Verification items for the finished model (mm, model axes). Give positions to 0.01 mm unless a question says otherwise; leave off trailing zeros. Loops run counter-clockwise (first coordinate to the right, second up) from the corner with the lowest first, then second, coordinate; pieces in that order, holes last. Notation, with made-up numbers: M -18,-5.75 L 16,-5.75 A11 ccw 16,1.25 Z; hole C 28,-8 d2. An arc over 180 degrees is marked long. Write each question's results on one line, items separated by ' | '. Start each with the question number.
```python
from build123d import *

# Parameters (mm, degrees)
F0_W     = 100
F0_H     = 200
F0_R     = 5.1
F0_W_2   = 70
F0_H_2   = 110
F0_H_3   = 15
F0_R_2   = 2.15
F1_DEPTH = 10
F2_R     = 5
F3_SIZE  = 1
F4_DEPTH = 5


with BuildPart() as f1:
    # F0 (on Top) → F1 (new body)
    with BuildSketch(Plane.XY):
        Rectangle(F0_W, F0_H)
        with Locations((-35, -90)):
            Circle(F0_R, mode=Mode.SUBTRACT)
        with Locations((35, -80)):
            Circle(F0_R, mode=Mode.SUBTRACT)
        with Locations((0, -15)):
            Rectangle(F0_W_2, F0_H_2, mode=Mode.SUBTRACT)
        with Locations((-35, 50)):
            Circle(F0_R, mode=Mode.SUBTRACT)
        with Locations((0, 77.5)):
            Rectangle(F0_W_2, F0_H_3, mode=Mode.SUBTRACT)
        with Locations((35, 60)):
            Circle(F0_R, mode=Mode.SUBTRACT)
        with Locations((35, -80)):
            Circle(F0_R)
        with Locations((35, -80)):
            Circle(F0_R_2, mode=Mode.SUBTRACT)
        with Locations((-35, -90)):
            Circle(F0_R)
        with Locations((-35, -90)):
            Circle(F0_R_2, mode=Mode.SUBTRACT)
        with Locations((-35, 50)):
            Circle(F0_R)
        with Locations((-35, 50)):
            Circle(F0_R_2, mode=Mode.SUBTRACT)
        with Locations((35, 60)):
            Circle(F0_R)
        with Locations((35, 60)):
            Circle(F0_R_2, mode=Mode.SUBTRACT)
    extrude(amount=F1_DEPTH)

    # F2
    f2_edges = [f1.edges().sort_by_distance(p)[0] for p in [
        (-50, -100, 5),
        (50, -100, 5),
        (35, -70, 5),
        (-35, -70, 5),
        (35, 40, 5),
        (-35, 40, 5),
        (-50, 100, 5),
        (50, 100, 5),
        (35, 70, 5),
        (35, 85, 5),
        (-35, 70, 5),
        (-35, 85, 5),
    ]]
    fillet(f2_edges, radius=F2_R)

    # F3
    f3_edges = [f1.edges().sort_by_distance(p)[0] for p in [
        (50, 0, 0),
        (48.535534, -98.535534, 0),
        (48.535534, 98.535534, 0),
        (0, -100, 0),
        (0, 100, 0),
        (-48.535534, -98.535534, 0),
        (-48.535534, 98.535534, 0),
        (-50, 0, 0),
        (32.85, -80, 0),
        (-37.15, -90, 0),
        (-37.15, 50, 0),
        (32.85, 60, 0),
        (0, -70, 0),
        (33.535534, -68.535534, 0),
        (-33.535534, -68.535534, 0),
        (35, -15, 0),
        (-35, -15, 0),
        (33.535534, 38.535534, 0),
        (-33.535534, 38.535534, 0),
        (0, 40, 0),
        (-35, 77.5, 0),
        (-33.535534, 71.464466, 0),
        (-33.535534, 83.535534, 0),
        (0, 70, 0),
        (0, 85, 0),
        (33.535534, 71.464466, 0),
        (33.535534, 83.535534, 0),
        (35, 77.5, 0),
    ]]
    chamfer(f3_edges, length=F3_SIZE)

    # F0 (on Top) → F4 (cut)
    with BuildSketch(Plane.XY):
        with Locations((-35, 50)):
            Circle(F0_R)
        with Locations((-35, 50)):
            Circle(F0_R_2, mode=Mode.SUBTRACT)
        with Locations((35, 60)):
            Circle(F0_R)
        with Locations((35, 60)):
            Circle(F0_R_2, mode=Mode.SUBTRACT)
        with Locations((35, -80)):
            Circle(F0_R)
        with Locations((35, -80)):
            Circle(F0_R_2, mode=Mode.SUBTRACT)
        with Locations((-35, -90)):
            Circle(F0_R)
        with Locations((-35, -90)):
            Circle(F0_R_2, mode=Mode.SUBTRACT)
    extrude(amount=F4_DEPTH, mode=Mode.SUBTRACT)


solid = f1.part
```
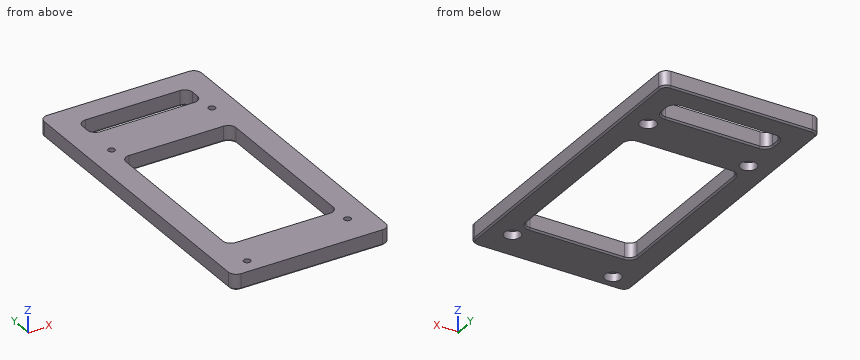
1. Depth check by flat-ended pin: pin 1 Ø16.5 at (x, y) = (35, 60) entering from -Z; pin 2 Ø5 at (x, y) = (-34, -88) entering from -Z; pin 3 Ø12 at (x, y) = (28.5, -2) entering from +Z. Enter the tip coordinate at first touch or a pass-through.
2. Thickness scan on probe 1 along Y at (x, z) = (-28, 4.75); probe 2 along X at (y, z) = (19.5, 1); probe 3 along Y at (x, z) = (36.5, 7). Record the ranges inside material, lowest first.
3. Section check B-B, the plane x = -19.5. Record the boundary of the cut face in (y, z), plus the area to 3 significant figures.
4. Section check A-A, the plane y = -13. Record the boundary of the cut face in (x, z), plus the area to 3 significant figures.
5. Section check C-C, the plane y = 60. Record the boundary of the cut face in (x, z).
Filled sheet:
1) pin 1: z = 0 | pin 2: z = 5 | pin 3: through
2) probe 1: -100 to -70, 40 to 70, 85 to 100 | probe 2: -50 to -35, 35 to 50 | probe 3: -100 to -81.54, -78.46 to 58.46, 61.54 to 100
3) outline: M -100,1 L -99,0 L -71,0 L -70,1 L -70,10 L -100,10 Z; M 40,1 L 41,0 L 69,0 L 70,1 L 70,10 L 40,10 Z; M 85,1 L 86,0 L 99,0 L 100,1 L 100,10 L 85,10 Z | area: 747 mm2
4) outline: M -50,1 L -49,0 L -36,0 L -35,1 L -35,10 L -50,10 Z; M 35,1 L 36,0 L 49,0 L 50,1 L 50,10 L 35,10 Z | area: 298 mm2
5) outline: M -50,1 L -49,0 L 29.9,0 L 29.9,5 L 32.85,5 L 32.85,10 L -50,10 Z; M 37.15,5 L 40.1,5 L 40.1,0 L 49,0 L 50,1 L 50,10 L 37.15,10 Z
